```python
from build123d import *

# Parameters (mm, degrees)
CROQUIS1_W              = 49.7
CROQUIS1_H              = 29.7
SALIENTE_EXTRUIR1_DEPTH = 1.5
CROQUIS2_R              = 5
SALIENTE_EXTRUIR2_DEPTH = 2
CROQUIS3_W              = 3
CROQUIS3_H              = 3
SALIENTE_EXTRUIR3_DEPTH = 1
CROQUIS4_W              = 3
CROQUIS4_H              = 1
SALIENTE_EXTRUIR4_DEPTH = 1.5
REDONDEO1_R             = 2
SALIENTE_EXTRUIR5_DEPTH = 5.75
CROQUIS7_R              = 1.5
CORTAR_EXTRUIR1_DEPTH   = 11.5


with BuildPart() as part:
    # Croquis1 → Saliente-Extruir1 (new body)
    with BuildSketch(Plane.XY):
        with Locations((0, 14.85)):
            Rectangle(CROQUIS1_W, CROQUIS1_H)
    extrude(amount=SALIENTE_EXTRUIR1_DEPTH)

    # Croquis2 → Saliente-Extruir2 (add)
    with BuildSketch(Plane.XY.offset(1.5)):
        with Locations((-13.85, 14.85)):
            Circle(CROQUIS2_R)
    extrude(amount=SALIENTE_EXTRUIR2_DEPTH)

    # Croquis3 → Saliente-Extruir3 (add)
    with BuildSketch(Plane.XY.offset(1.5)):
        with Locations((-22.85, 1.5)):
            Rectangle(CROQUIS3_W, CROQUIS3_H)
        with Locations((22.85, 1.5)):
            Rectangle(CROQUIS3_W, CROQUIS3_H)
    extrude(amount=SALIENTE_EXTRUIR3_DEPTH)

    # Croquis4 → Saliente-Extruir4 (add)
    with BuildSketch(Plane.XZ):
        with Locations((-22.85, 2)):
            Rectangle(CROQUIS4_W, CROQUIS4_H)
        with Locations((22.85, 2)):
            Rectangle(CROQUIS4_W, CROQUIS4_H)
    extrude(amount=SALIENTE_EXTRUIR4_DEPTH)

    # Redondeo1
    # the kernel refuses this fillet: 2 mm, written as the material it takes off along each edge
    with BuildSketch(Plane(origin=(-17.019872981, 3, 2.5), x_dir=(0, -1, 0), z_dir=(-1, 0, 0)), Plane(origin=(28.680127019, 3, 2.5), x_dir=(0, -1, 0), z_dir=(-1, 0, 0))) as redondeo1_piece_1:
        with BuildLine():
            CenterArc((1.732050808, -2), REDONDEO1_R, 90, 60)
            Line((0, -1), (-0.034641016, -0.98))
            ThreePointArc((-0.034641016, -0.98), (-0.04, -0.5), (-0.04, 0))
            Line((-0.04, 0), (0, 0.04))
            Line((0, 0.04), (1.732050808, 0.04))
            Line((1.732050808, 0.04), (1.732050808, 0))
        make_face()
    extrude(amount=11.660254038, mode=Mode.SUBTRACT)

    # Croquis6 → Saliente-Extruir5 (add, symmetric)
    with BuildSketch(Plane(origin=(0, 0, 0), x_dir=(0, 0, -1), z_dir=(1, 0, 0))):
        with BuildLine():
            Line((0, 29.7), (-6.265388986, 29.7))
            ThreePointArc((-6.265388986, 29.7), (-7.234013908, 30.451472819), (-6.746848229, 31.57646848))
            Line((-6.746848229, 31.57646848), (0, 35.282628504))
            Line((0, 35.282628504), (0, 34.141686163))
            Line((0, 34.141686163), (-4.557388257, 31.63823424))
            ThreePointArc((-4.557388257, 31.63823424), (-4.800971096, 31.075736409), (-4.316658635, 30.7))
            Line((-4.316658635, 30.7), (0, 30.7))
            Line((0, 30.7), (0, 29.7))
        make_face()
    extrude(amount=SALIENTE_EXTRUIR5_DEPTH, both=True)

    # Croquis7 → Cortar-Extruir1 (cut)
    with BuildSketch(Plane(origin=(0, 0, 0), x_dir=(-1, 0, 0), z_dir=(0, 0, -1))):
        with Locations((0, 25)):
            Circle(CROQUIS7_R)
    extrude(amount=-CORTAR_EXTRUIR1_DEPTH, mode=Mode.SUBTRACT)


solid = part.part
```
Design review of the part built by this model. Coordinates are the model's own, in mm. A direction names the side the tool comes from. Give positions to 0.01 mm unless a question says otherwise; leave off trailing zeros. Write each loop counter-clockwise with the first axis right and the second up, starting at its lowest first coordinate (ties: lowest second). Pieces come first, ordered by that corner, then holes. Notation, with made-up numbers: (-3.5, 70.5) -> (37.5, 70.5) arc R14 cw to (37.5, 96.5) -> close; hole circle Ø3 at (21, -38.75). An arc over 180 degrees is marked (long way). Answer in a Markdown table with one row per item.
(1) To check wall thickness, follow probe 1 along Y at (x, z) = (0, 0.65); probe 2 along Z at (x, y) = (13.5, 18); probe 3 along Y at (x, z) = (0, 1.05). State the ranges of each line that lie inside material, in increasing order.
Results:
| item | result |
|---|---|
| probe 1 | 0 to 23.5, 26.5 to 30.7, 33.78 to 34.93 |
| probe 2 | 0 to 1.5 |
| probe 3 | 0 to 23.5, 26.5 to 30.7, 33.56 to 34.71 |
(2) Mouldability with a two-part tool opening along X and no side actions: class faces 1 (the flat face through (-24.35, 1, 2)), 2 (the cylindrical face through (0.195, 26.487, 0.74)), 3 (the flat face through (21.35, 1, 2)), 4 (the cylindrical face through (-11.162, 19.066, 2.486)) as +X half, -X half, draft (parallel to the pull), parting line (faces both ways), or undercut.
Results:
| item | result |
|---|---|
| face 1 | -X half |
| face 2 | undercut |
| face 3 | undercut |
| face 4 | parting line |
(3) Consider section C-C (y = 14.85). State the section outline as (x, z) points, then the cut area to 4 significant figures.
Results:
| item | result |
|---|---|
| outline | (-24.85, 0) -> (24.85, 0) -> (24.85, 1.5) -> (-8.85, 1.5) -> (-8.85, 3.5) -> (-18.85, 3.5) -> (-18.85, 1.5) -> (-24.85, 1.5) -> close |
| area | 94.55 mm2 |
(4) Consider section D-D (x = -13.85). State the section outline as (y, z) points, then the cut area to 4 significant figures.
Results:
| item | result |
|---|---|
| outline | (0, 0) -> (29.7, 0) -> (29.7, 1.5) -> (19.85, 1.5) -> (19.85, 3.5) -> (9.85, 3.5) -> (9.85, 1.5) -> (0, 1.5) -> close |
| area | 64.55 mm2 |
(5) For faces 5 (the flat face through (0, 0, 1)), 6 (the flat face through (0, 15, 1.5)), 7 (the flat face through (0, 30.7, 2)), 8 (the flat face through (-21.35, 1, 2)), 9 (the flat face through (15, 29.7, 1)), list the 3-axis set-ups (+Z, -Z, +X, -X, +Y, -Y) from which the entire face can be reached by the end or side of a thin tool; tool diameter is ignored.
Results:
| item | result |
|---|---|
| face 5 | -Z, +X, -X, -Y |
| face 6 | +Z |
| face 7 | -Z, +X, -X |
| face 8 | +Z, +Y, -Y |
| face 9 | +Z, -Z, +X, +Y |
(6) Consider section A-A (y = 25). State the section outline as (x, z) points.
Results:
| item | result |
|---|---|
| outline | (-24.85, 0) -> (-1.5, 0) -> (-1.5, 1.5) -> (-24.85, 1.5) -> close; (1.5, 0) -> (24.85, 0) -> (24.85, 1.5) -> (1.5, 1.5) -> close |
(7) Clearance check with flat-ended pins moving along their axes: pin 1 (2 mm diameter, centred on x = 0.5, z = 2.5, fed in from +Y); pin 2 (1.1 mm diameter, centred on y = 1, z = 2, fed in from +X); pin 3 (5 mm diameter, centred on x = 0, y = 25, fed in from +Z); pin 4 (1.2 mm diameter, centred on x = 23.5, y = -1, fed in from -Z). State where each tip first meets the part, or that it passes through.
Results:
| item | result |
|---|---|
| pin 1 | y = 34.46 |
| pin 2 | x = 24.85 |
| pin 3 | z = 1.5 |
| pin 4 | z = 1.5 |
(8) Consider section B-B (x = 0). State the section outline as (y, z) points, then the cut area to 3 significant figures.
Results:
| item | result |
|---|---|
| outline | (0, 0) -> (23.5, 0) -> (23.5, 1.5) -> (0, 1.5) -> close; (26.5, 0) -> (30.7, 0) -> (30.7, 4.32) arc R0.5 cw to (31.64, 4.56) -> (34.14, 0) -> (35.28, 0) -> (31.58, 6.75) arc R1 ccw to (29.7, 6.27) -> (29.7, 1.5) -> (26.5, 1.5) -> close |
| area | 55.7 mm2 |
